from build123d import *

# Parameters (mm, degrees)
BOSS_EXTRUDE1_DEPTH      = 61.14
SKETCH2_R                = 80
BOSS_EXTRUDE2_DEPTH      = 2
SKETCH3_R                = 83
SKETCH3_R_2              = 80
BOSS_EXTRUDE3_DEPTH      = 49.01
SKETCH6_R                = 83
SKETCH6_R_2              = 32.5
BOSS_EXTRUDE4_DEPTH      = 2
MOVE_START               = -80.2
MOVE_FACE1_OUTLINE_W     = 61.14
MOVE_FACE1_OUTLINE_H     = 0.2
MOVE_FACE1_DEPTH         = 160.4
MOVE_FACE1_2_OUTLINE_R   = 80.2
MOVE_FACE1_2_OUTLINE_R_2 = 80
MOVE_FACE1_2_DEPTH       = 112.15
MOVE_FACE1_3_DEPTH       = 61.14
SKETCH7_R                = 5
CUT_EXTRUDE1_DEPTH       = 164.732166968
CUT_EXTRUDE2_DEPTH       = 216.762514121


with BuildPart() as part:
    # Sketch1 → Boss-Extrude1 (new body)
    with BuildSketch(Plane(origin=(0, 0, 0), x_dir=(1, 0, 0), z_dir=(0, 1, 0))):
        with BuildLine():
            Line((0, -83), (83, -83))
            Line((83, -83), (83, 0))
            ThreePointArc((83, 0), (0, 83), (-83, 0))
            Line((-83, 0), (-83, -83))
            Line((-83, -83), (0, -83))
        make_face()
        with BuildLine():
            Line((-80, 0), (-80, -80))
            Line((-80, -80), (0, -80))
            Line((0, -80), (80, -80))
            Line((80, -80), (80, 0))
            ThreePointArc((80, 0), (0, 80), (-80, 0))
        make_face(mode=Mode.SUBTRACT)
    extrude(amount=BOSS_EXTRUDE1_DEPTH)

    # Sketch2 → Boss-Extrude2 (add)
    with BuildSketch(Plane(origin=(0, 61.14, 0), x_dir=(1, 0, 0), z_dir=(0, 1, 0))):
        with BuildLine():
            Line((-83, -83), (83, -83))
            Line((83, -83), (83, 0))
            ThreePointArc((83, 0), (0, 83), (-83, 0))
            Line((-83, 0), (-83, -83))
        make_face()
        with Locations(Location((0, 0, 0), (0, 0, 270))):
            Circle(SKETCH2_R, mode=Mode.SUBTRACT)
    extrude(amount=BOSS_EXTRUDE2_DEPTH)

    # Sketch3 → Boss-Extrude3 (add)
    with BuildSketch(Plane(origin=(0, 63.14, 0), x_dir=(1, 0, 0), z_dir=(0, 1, 0))):
        with Locations(Location((0, 0, 0), (0, 0, 270))):
            Circle(SKETCH3_R)
        with Locations(Location((0, 0, 0), (0, 0, 270))):
            Circle(SKETCH3_R_2, mode=Mode.SUBTRACT)
    extrude(amount=BOSS_EXTRUDE3_DEPTH)

    # Sketch6 → Boss-Extrude4 (add)
    with BuildSketch(Plane(origin=(0, 112.15, 0), x_dir=(1, 0, 0), z_dir=(0, 1, 0))):
        with Locations(Location((0, 0, 0), (0, 0, 270))):
            Circle(SKETCH6_R)
        with Locations(Location((0, 0, 0), (0, 0, 270))):
            Circle(SKETCH6_R_2, mode=Mode.SUBTRACT)
    extrude(amount=BOSS_EXTRUDE4_DEPTH)

    # Move Face1: read off the stored shape, not the designer's step
    # Move Face1 outline → Move Face1 (cut)
    with BuildSketch(Plane.YZ.offset(MOVE_START)):
        with Locations((30.57, 80.1)):
            Rectangle(MOVE_FACE1_OUTLINE_W, MOVE_FACE1_OUTLINE_H)
    extrude(amount=MOVE_FACE1_DEPTH, mode=Mode.SUBTRACT)

    # Move Face1 2 outline → Move Face1 2 (cut)
    with BuildSketch(Plane(origin=(0, 0, 0), x_dir=(1, 0, 0), z_dir=(0, 1, 0))):
        Circle(MOVE_FACE1_2_OUTLINE_R)
        Circle(MOVE_FACE1_2_OUTLINE_R_2, mode=Mode.SUBTRACT)
    extrude(amount=MOVE_FACE1_2_DEPTH, mode=Mode.SUBTRACT)

    # Move Face1 3 outline → Move Face1 3 (cut)
    with BuildSketch(Plane(origin=(0, 0, 0), x_dir=(1, 0, 0), z_dir=(0, 1, 0))):
        with BuildLine():
            Line((80.2, -80), (80.2, 0))
            ThreePointArc((80.2, 0), (80.149984404, -2.831960452), (80, -5.660388679))
            Line((80, -5.660388679), (80, -80))
            Line((80, -80), (80.2, -80))
        make_face()
        with BuildLine():
            ThreePointArc((-80, -5.660388679), (-80.149984404, -2.831960452), (-80.2, 0))
            Line((-80.2, 0), (-80.2, -80))
            Line((-80.2, -80), (-80, -80))
            Line((-80, -80), (-80, -5.660388679))
        make_face()
    extrude(amount=MOVE_FACE1_3_DEPTH, mode=Mode.SUBTRACT)

    # Sketch7 → Cut-Extrude1 (cut, through all)
    with BuildSketch(Plane(origin=(0, 114.15, 0), x_dir=(1, 0, 0), z_dir=(0, 1, 0))):
        with Locations(Location((0, 73, 0), (0, 0, 270))):
            Circle(SKETCH7_R)
        with Locations(Location((73, 0, 0), (0, 0, 270))):
            Circle(SKETCH7_R)
        with Locations(Location((0, -73, 0), (0, 0, 270))):
            Circle(SKETCH7_R)
        with Locations(Location((-73, 0, 0), (0, 0, 270))):
            Circle(SKETCH7_R)
    extrude(amount=-CUT_EXTRUDE1_DEPTH, mode=Mode.SUBTRACT)

    # Sketch8 → Cut-Extrude2 (cut, through all)
    with BuildSketch(Plane(origin=(0, 0, 80.2), x_dir=(-1, 0, 0), z_dir=(0, 0, -1))):
        Polygon((-80.2, 0), (80.2, 0), (80.2, 61.14), (0, 61.14), (-80.2, 61.14), align=None)
    extrude(amount=-CUT_EXTRUDE2_DEPTH, mode=Mode.SUBTRACT)


solid = part.part
Geometry: final body of the model. Coordinates: model frame, mm. A direction names the side the tool comes from. Coordinates: 2 decimals unless noted, no trailing zeros. Order: outer loops, then holes, each group sorted by start corner. A loop starts at its lowest first (then second) coordinate and runs counter-clockwise, first axis right, second up.
1) First-contact query: P1, Ø6, axis at x = -3, z = 33.5, coming from the -Y side; P2, Ø1.5, axis at y = 101, z = -50, coming from the +X side; P3, Ø4, axis at y = 93.5, z = -53, coming from the -X side; P4, Ø16, axis at x = 0, z = -73, coming from the -Y side. Flat tips, straight axial feed; report the tip coordinate or a pass-through.
Result sheet:
P1: stops at y = 112.15
P2: stops at x = 66.81
P3: stops at x = -65.48
P4: stops at y = 0
2) Ray query, probe 1 along X at (y, z) = (56, 5); probe 2 along Y at (x, z) = (22, 27). Return the intervals inside material, ascending.
Result sheet:
probe 1: x = -83 to -80.2, 80.2 to 83
probe 2: y = 112.15 to 114.15
3) Section C-C (y = 39). Return loops of the section in (x, z).
Result sheet:
outline: (-83, 0) arc R83 ccw to (83, 0) - (83, 83) - (80.2, 83) - (80.2, 0) arc R80.2 cw to (-80.2, 0) - (-80.2, 83) - (-83, 83) - close
4) Section B-B (z = -73). Return loops of the section in (x, y), then the cut area to 3 significant figures.
Result sheet:
outline: (-39.5, 0) - (-33.21, 0) - (-33.21, 112.15) - (-5, 112.15) - (-5, 114.15) - (-39.5, 114.15) - close; (5, 112.15) - (33.21, 112.15) - (33.21, 0) - (39.5, 0) - (39.5, 114.15) - (5, 114.15) - close
area: 1,550 mm2
5) Draft query along Z for faces 1 (the flat face through (-37, 62, 83)), 2 (the cylindrical face through (-77.88, 113.16, -1.08)), 3 (the flat face through (80.2, 31, 41)). Return one class per face: released by +Z, released by -Z, zero draft, split by the parting line, or undercut.
Result sheet:
face 1: released by +Z
face 2: undercut
face 3: zero draft
6) Set-up query: faces 4 (the cylindrical face through (-10.44, 67.751, -79.518)), 5 (the cylindrical face through (3.65, 68.96, -82.92)), 6 (the flat face through (-66, 63.14, 63)), 7 (the flat face through (66, 63.14, 66)), 8 (the flat face through (0, 61.14, 81)). Return all of +Z, -Z, +X, -X, +Y, -Y with unobstructed straight access to the full face (end or side cutting, diameter ignored); none if empty.
Result sheet:
face 4: -Y
face 5: +Y
face 6: +Z, -X, +Y
face 7: +Z, +X, +Y
face 8: +Z, -Y
7) Section D-D (x = 43). Return loops of the section in (y, z).
Result sheet:
outline: (0, -70.99) - (114.15, -70.99) - (114.15, 70.99) - (63.14, 70.99) - (63.14, 83) - (61.14, 83) - (61.14, 67.7) - (112.15, 67.7) - (112.15, -67.7) - (0, -67.7) - close
8) Section A-A (x = 18.5). Return loops of the section in (y, z), then the cut area to 3 significant figures.
Result sheet:
outline: (0, -80.91) - (114.15, -80.91) - (114.15, -26.72) - (112.15, -26.72) - (112.15, -78.04) - (0, -78.04) - close; (61.14, 78.04) - (112.15, 78.04) - (112.15, 26.72) - (114.15, 26.72) - (114.15, 80.91) - (63.14, 80.91) - (63.14, 83) - (61.14, 83) - close
area: 690 mm2
